from build123d import *

# Parameters (mm, degrees)
ESQUISSE1_R                  = 1.8
BOSS_EXTRU_1_DEPTH           = 1
ESQUISSE2_R                  = 1.5
BOSS_EXTRU_2_DEPTH           = 3
ESQUISSE4_R                  = 0.149962486
BOSS_EXTRU_3_DEPTH           = 3
R_P_TITION_CIRCULAIRE1_COUNT = 2


with BuildPart() as part:
    # Esquisse1 → Boss.-Extru.1 (new body)
    with BuildSketch(Plane.XY):
        Circle(ESQUISSE1_R)
    extrude(amount=BOSS_EXTRU_1_DEPTH)

    # Esquisse2 → Boss.-Extru.2 (add)
    with BuildSketch(Plane.XY.offset(1)):
        Circle(ESQUISSE2_R)
    extrude(amount=BOSS_EXTRU_2_DEPTH)

    # Esquisse4 → Boss.-Extru.3 (add)
    with BuildSketch(Plane(origin=(0, 0, 0), x_dir=(-1, 0, 0), z_dir=(0, 0, -1))):
        with Locations(Location((0, -0.732458838, 0), (0, 0, 180))):
            Circle(ESQUISSE4_R)
    boss_extru_3 = extrude(amount=BOSS_EXTRU_3_DEPTH)

    # Esquisse3 → R_volution7 (revolve)
    with BuildSketch(Plane(origin=(0, 0, 0), x_dir=(1, 0, 0), z_dir=(0, 1, 0))):
        with BuildLine():
            Line((-1.5, -4), (0, -4))
            Line((0, -4), (0, -5.5))
            ThreePointArc((0, -5.5), (-1.060660172, -5.060660172), (-1.5, -4))
        make_face()
    revolve(axis=Axis((0, 0, -0.275), (0, 0, 1)))

    # R_p_tition circulaire1: Boss.-Extru.3 ×2 about axis
    r_p_tition_circulaire1_axis = Axis((0, 0, 0), (0, 0, 1))
    for i in range(1, R_P_TITION_CIRCULAIRE1_COUNT):
        add(boss_extru_3.rotate(r_p_tition_circulaire1_axis, i * 360 / R_P_TITION_CIRCULAIRE1_COUNT))


solid = part.part
Input: part model. Units: mm. Frame: model coordinates. A direction names the side the tool comes from. Give positions to 0.01 mm unless a question says otherwise; leave off trailing zeros. Loops run counter-clockwise (first coordinate to the right, second up) from the corner with the lowest first, then second, coordinate; pieces in that order, holes last. Notation, with made-up numbers: (-37, -1) -> (-11, -1) arc R24 cw to (-11, 12) -> close; hole circle Ø10 at (-36, -17). An arc over 180 degrees is marked (long way). Answer as a JSON object with one key per item and string values. Group by question number.
Item 1: Cut plane D-D, the plane x = -1.3. Return the cut outline in (y, z), and give its area (3 significant figures).
Item 2: Reachability of faces 1 (the cylindrical face through (1.717, 0.541, 0.493)), 2 (the cylindrical face through (-1.5, 0.07, 2.48)) from +Z, -Z, +X, -X, +Y, -Y: full face, straight path, thin tool, end or side. Return the list, or none.
Item 3: Cut plane B-B, the plane y = 0. Return the cut outline in (x, z).
Item 4: Line query: probe 1 along Z at (x, y) = (1.45, 0.5); probe 2 along Y at (x, z) = (-0.15, 4); probe 3 along X at (y, z) = (0.45, 3). Output: solid intervals per line, ascending.
Item 5: Pin query (flat end, axial travel): P1, Ø1, axis at y = 1, z = -2, coming from the -X side. Return the tip coordinate at first contact, or that it passes through.
Item 6: Cut plane A-A, the plane x = 0. Return the cut outline in (y, z).
Item 7: Cut plane C-C, the plane z = 1.75. Return the cut outline in (x, y), and give its area (3 significant figures).
Checks:
{
 "1": {"outline": "(-1.24, 0) -> (1.24, 0) -> (1.24, 1) -> (0.75, 1) -> (0.75, 4) arc R0.75 ccw to (-0.75, 4) -> (-0.75, 1) -> (-1.24, 1) -> close", "area": "7.86 mm²"},
 "2": {"face 1": "+Z, -Z", "face 2": "+Z"},
 "3": {"outline": "(-1.8, 0) -> (1.8, 0) -> (1.8, 1) -> (1.5, 1) -> (1.5, 4) arc R1.5 ccw to (-1.5, 4) -> (-1.5, 1) -> (-1.8, 1) -> close"},
 "4": {"probe 1": "z = 0 to 1", "probe 2": "y = -1.49 to 1.49", "probe 3": "x = -1.43 to 1.43"},
 "5": {"P1": "stops at x = -0.15"},
 "6": {"outline": "(-1.8, 0) -> (-0.88, 0) -> (-0.88, -3) -> (-0.58, -3) -> (-0.58, 0) -> (0.58, 0) -> (0.58, -3) -> (0.88, -3) -> (0.88, 0) -> (1.8, 0) -> (1.8, 1) -> (1.5, 1) -> (1.5, 4) arc R1.5 ccw to (-1.5, 4) -> (-1.5, 1) -> (-1.8, 1) -> close"},
 "7": {"outline": "circle Ø3 at (0, 0)", "area": "7.07 mm²"}
}
